```python
from build123d import *

# Parameters (mm, degrees)
SKETCH1_W                      = 300
SKETCH1_H                      = 350
BASE_FLANGE1_DEPTH             = 0.9
EDGE_FLANGE1_STRIP_W           = 5.4
EDGE_FLANGE1_STRIP_H           = 0.9
EDGE_FLANGE1_STRIP_CUT_DEPTH   = 350
EDGE_FLANGE1_STRIP_2_W         = 5.4
EDGE_FLANGE1_STRIP_2_H         = 0.9
EDGE_FLANGE1_STRIP_CUT_2_DEPTH = 350
EDGE_FLANGE1_DEPTH             = 350
EDGE_FLANGE1_BEND_DEPTH        = 350
EDGE_FLANGE2_STRIP_W           = 5.4
EDGE_FLANGE2_STRIP_H           = 0.9
EDGE_FLANGE2_STRIP_CUT_DEPTH   = 350
EDGE_FLANGE2_STRIP_2_W         = 5.4
EDGE_FLANGE2_STRIP_2_H         = 0.9
EDGE_FLANGE2_STRIP_CUT_2_DEPTH = 350
EDGE_FLANGE2_DEPTH             = 350
EDGE_FLANGE2_BEND_DEPTH        = 350
EDGE_FLANGE3_STRIP_W           = 5.4
EDGE_FLANGE3_STRIP_H           = 0.9
EDGE_FLANGE3_STRIP_CUT_DEPTH   = 350
EDGE_FLANGE3_STRIP_2_W         = 5.4
EDGE_FLANGE3_STRIP_2_H         = 0.9
EDGE_FLANGE3_STRIP_CUT_2_DEPTH = 350
EDGE_FLANGE3_DEPTH             = 350
EDGE_FLANGE3_BEND_DEPTH        = 350
CUT_EXTRUDE1_START             = 160
CUT_EXTRUDE1_DEPTH             = 15
MIRROR2_START                  = 160
MIRROR2_COPY_1_DEPTH           = 15
EDGE_FLANGE4_STRIP_W           = 5.4
EDGE_FLANGE4_STRIP_H           = 0.9
EDGE_FLANGE4_STRIP_CUT_DEPTH   = 320
EDGE_FLANGE4_DEPTH             = 320
SKETCH28_R                     = 3
CUT_EXTRUDE2_DEPTH             = 10


# Read off the part's stored shape, not the designer's step: Cut-Extrude1
# Sheet-metal steps are written as plain solids
with BuildPart() as part:
    # Sketch1 → Base-Flange1 (new body)
    with BuildSketch(Plane.XY):
        Rectangle(SKETCH1_W, SKETCH1_H)
    extrude(amount=-BASE_FLANGE1_DEPTH)

    # Edge-Flange1 strip (across the edge) → Edge-Flange1 strip cut (cut)
    with BuildSketch(Plane(origin=(-150, 175, 0), x_dir=(1, 0, 0), z_dir=(0, -1, 0))):
        with Locations((-0.9, -0.45)):
            Rectangle(EDGE_FLANGE1_STRIP_W, EDGE_FLANGE1_STRIP_H)
    extrude(amount=EDGE_FLANGE1_STRIP_CUT_DEPTH, mode=Mode.SUBTRACT)

    # Edge-Flange1 strip 2 (across the edge) → Edge-Flange1 strip cut 2 (cut)
    with BuildSketch(Plane(origin=(150, -175, 0), x_dir=(-1, 0, 0), z_dir=(0, 1, 0))):
        with Locations((-0.9, -0.45)):
            Rectangle(EDGE_FLANGE1_STRIP_2_W, EDGE_FLANGE1_STRIP_2_H)
    extrude(amount=EDGE_FLANGE1_STRIP_CUT_2_DEPTH, mode=Mode.SUBTRACT)

    # Edge-Flange1 section (across the edge) → Edge-Flange1 (add)
    with BuildSketch(Plane(origin=(-150, 175, 0), x_dir=(1, 0, 0), z_dir=(0, -1, 0))):
        with BuildLine():
            Line((0, 0.9), (0, 199.1))
            Line((0, 199.1), (0.9, 199.1))
            Line((0.9, 199.1), (0.9, 0.9))
            ThreePointArc((0.9, 0.9), (1.163603897, 0.263603897), (1.8, 0))
            Line((1.8, 0), (1.8, -0.9))
            ThreePointArc((1.8, -0.9), (0.527207794, -0.372792206), (0, 0.9))
        make_face()
    extrude(amount=EDGE_FLANGE1_DEPTH)

    # Edge-Flange1 section 2 (across the edge) → Edge-Flange1 bend (add)
    with BuildSketch(Plane(origin=(150, -175, 0), x_dir=(-1, 0, 0), z_dir=(0, 1, 0))):
        with BuildLine():
            Line((0, 0.9), (0, 199.1))
            Line((0, 199.1), (0.9, 199.1))
            Line((0.9, 199.1), (0.9, 0.9))
            ThreePointArc((0.9, 0.9), (1.163603897, 0.263603897), (1.8, 0))
            Line((1.8, 0), (1.8, -0.9))
            ThreePointArc((1.8, -0.9), (0.527207794, -0.372792206), (0, 0.9))
        make_face()
    extrude(amount=EDGE_FLANGE1_BEND_DEPTH)

    # Edge-Flange2 strip (across the edge) → Edge-Flange2 strip cut (cut)
    with BuildSketch(Plane(origin=(-149.1, 175, 199.1), x_dir=(0, 0, -1), z_dir=(0, -1, 0))):
        with Locations((-0.9, -0.45)):
            Rectangle(EDGE_FLANGE2_STRIP_W, EDGE_FLANGE2_STRIP_H)
    extrude(amount=EDGE_FLANGE2_STRIP_CUT_DEPTH, mode=Mode.SUBTRACT)

    # Edge-Flange2 strip 2 (across the edge) → Edge-Flange2 strip cut 2 (cut)
    with BuildSketch(Plane(origin=(149.1, -175, 199.1), x_dir=(0, 0, -1), z_dir=(0, 1, 0))):
        with Locations((-0.9, -0.45)):
            Rectangle(EDGE_FLANGE2_STRIP_2_W, EDGE_FLANGE2_STRIP_2_H)
    extrude(amount=EDGE_FLANGE2_STRIP_CUT_2_DEPTH, mode=Mode.SUBTRACT)

    # Edge-Flange2 section (across the edge) → Edge-Flange2 (add)
    with BuildSketch(Plane(origin=(-149.1, 175, 199.1), x_dir=(0, 0, -1), z_dir=(0, -1, 0))):
        with BuildLine():
            Line((0, 0.9), (0, 19.1))
            Line((0, 19.1), (0.9, 19.1))
            Line((0.9, 19.1), (0.9, 0.9))
            ThreePointArc((0.9, 0.9), (1.163603897, 0.263603897), (1.8, 0))
            Line((1.8, 0), (1.8, -0.9))
            ThreePointArc((1.8, -0.9), (0.527207794, -0.372792206), (0, 0.9))
        make_face()
    extrude(amount=EDGE_FLANGE2_DEPTH)

    # Edge-Flange2 section 2 (across the edge) → Edge-Flange2 bend (add)
    with BuildSketch(Plane(origin=(149.1, -175, 199.1), x_dir=(0, 0, -1), z_dir=(0, 1, 0))):
        with BuildLine():
            Line((0, 0.9), (0, 19.1))
            Line((0, 19.1), (0.9, 19.1))
            Line((0.9, 19.1), (0.9, 0.9))
            ThreePointArc((0.9, 0.9), (1.163603897, 0.263603897), (1.8, 0))
            Line((1.8, 0), (1.8, -0.9))
            ThreePointArc((1.8, -0.9), (0.527207794, -0.372792206), (0, 0.9))
        make_face()
    extrude(amount=EDGE_FLANGE2_BEND_DEPTH)

    # Edge-Flange3 strip (across the edge) → Edge-Flange3 strip cut (cut)
    with BuildSketch(Plane(origin=(130, -175, 198.2), x_dir=(1, 0, 0), z_dir=(0, 1, 0))):
        with Locations((-0.9, -0.45)):
            Rectangle(EDGE_FLANGE3_STRIP_W, EDGE_FLANGE3_STRIP_H)
    extrude(amount=EDGE_FLANGE3_STRIP_CUT_DEPTH, mode=Mode.SUBTRACT)

    # Edge-Flange3 strip 2 (across the edge) → Edge-Flange3 strip cut 2 (cut)
    with BuildSketch(Plane(origin=(-130, 175, 198.2), x_dir=(-1, 0, 0), z_dir=(0, -1, 0))):
        with Locations((-0.9, -0.45)):
            Rectangle(EDGE_FLANGE3_STRIP_2_W, EDGE_FLANGE3_STRIP_2_H)
    extrude(amount=EDGE_FLANGE3_STRIP_CUT_2_DEPTH, mode=Mode.SUBTRACT)

    # Edge-Flange3 section (across the edge) → Edge-Flange3 (add)
    with BuildSketch(Plane(origin=(130, -175, 198.2), x_dir=(1, 0, 0), z_dir=(0, 1, 0))):
        with BuildLine():
            Line((0, 0.9), (0, 19.1))
            Line((0, 19.1), (0.9, 19.1))
            Line((0.9, 19.1), (0.9, 0.9))
            ThreePointArc((0.9, 0.9), (1.163603897, 0.263603897), (1.8, 0))
            Line((1.8, 0), (1.8, -0.9))
            ThreePointArc((1.8, -0.9), (0.527207794, -0.372792206), (0, 0.9))
        make_face()
    extrude(amount=EDGE_FLANGE3_DEPTH)

    # Edge-Flange3 section 2 (across the edge) → Edge-Flange3 bend (add)
    with BuildSketch(Plane(origin=(-130, 175, 198.2), x_dir=(-1, 0, 0), z_dir=(0, -1, 0))):
        with BuildLine():
            Line((0, 0.9), (0, 19.1))
            Line((0, 19.1), (0.9, 19.1))
            Line((0.9, 19.1), (0.9, 0.9))
            ThreePointArc((0.9, 0.9), (1.163603897, 0.263603897), (1.8, 0))
            Line((1.8, 0), (1.8, -0.9))
            ThreePointArc((1.8, -0.9), (0.527207794, -0.372792206), (0, 0.9))
        make_face()
    extrude(amount=EDGE_FLANGE3_BEND_DEPTH)

    # Cut-Extrude1 outline → Cut-Extrude1 (cut)
    with BuildSketch(Plane(origin=(0, 0, 0), x_dir=(1, 0, 0), z_dir=(0, 1, 0)).offset(CUT_EXTRUDE1_START)):
        with BuildLine():
            ThreePointArc((-148.2, -198.2), (-148.836396103, -197.936396103), (-149.1, -197.3))
            Line((-149.1, -197.3), (-150, -197.3))
            ThreePointArc((-150, -197.3), (-149.472792206, -198.572792206), (-148.2, -199.1))
            Line((-148.2, -199.1), (-131.8, -199.1))
            ThreePointArc((-131.8, -199.1), (-130.527207794, -198.572792206), (-130, -197.3))
            Line((-130, -197.3), (-130, -179.1))
            Line((-130, -179.1), (-130.9, -179.1))
            Line((-130.9, -179.1), (-130.9, -197.3))
            ThreePointArc((-130.9, -197.3), (-131.163603897, -197.936396103), (-131.8, -198.2))
            Line((-131.8, -198.2), (-148.2, -198.2))
        make_face()
    cut_extrude1 = extrude(amount=CUT_EXTRUDE1_DEPTH, mode=Mode.SUBTRACT)

    # Mirror1: Cut-Extrude1 across plane
    add(cut_extrude1.mirror(Plane(origin=(0, 0, 0), x_dir=(0, 0, 1), z_dir=(1, 0, 0))), mode=Mode.SUBTRACT)

    # Mirror2: Cut-Extrude1 across plane
    add(cut_extrude1.mirror(Plane.ZX), mode=Mode.SUBTRACT)

    # Mirror2 copy 1 sketch → Mirror2 copy 1 (cut)
    with BuildSketch(Plane(origin=(0, 0, 0), x_dir=(-1, 0, 0), z_dir=(0, -1, 0)).offset(MIRROR2_START)):
        with BuildLine():
            ThreePointArc((-148.2, -198.2), (-148.836396103, -197.936396103), (-149.1, -197.3))
            Line((-149.1, -197.3), (-150, -197.3))
            ThreePointArc((-150, -197.3), (-149.472792206, -198.572792206), (-148.2, -199.1))
            Line((-148.2, -199.1), (-131.8, -199.1))
            ThreePointArc((-131.8, -199.1), (-130.527207794, -198.572792206), (-130, -197.3))
            Line((-130, -197.3), (-130, -179.1))
            Line((-130, -179.1), (-130.9, -179.1))
            Line((-130.9, -179.1), (-130.9, -197.3))
            ThreePointArc((-130.9, -197.3), (-131.163603897, -197.936396103), (-131.8, -198.2))
            Line((-131.8, -198.2), (-148.2, -198.2))
        make_face()
    extrude(amount=MIRROR2_COPY_1_DEPTH, mode=Mode.SUBTRACT)

    # Edge-Flange4 strip (across the edge) → Edge-Flange4 strip cut (cut)
    with BuildSketch(Plane(origin=(130, 160, 179.1), x_dir=(0, 0, 1), z_dir=(0, -1, 0))):
        with Locations((-1.8, -0.45)):
            Rectangle(EDGE_FLANGE4_STRIP_W, EDGE_FLANGE4_STRIP_H)
    extrude(amount=EDGE_FLANGE4_STRIP_CUT_DEPTH, mode=Mode.SUBTRACT)

    # Edge-Flange4 section (across the edge) → Edge-Flange4 (add)
    with BuildSketch(Plane(origin=(130, 160, 179.1), x_dir=(0, 0, 1), z_dir=(0, -1, 0))):
        with BuildLine():
            Line((-0.9, 0.9), (-0.9, 14.1))
            Line((-0.9, 14.1), (0, 14.1))
            Line((0, 14.1), (0, 0.9))
            ThreePointArc((0, 0.9), (0.263603897, 0.263603897), (0.9, 0))
            Line((0.9, 0), (0.9, -0.9))
            ThreePointArc((0.9, -0.9), (-0.372792206, -0.372792206), (-0.9, 0.9))
        make_face()
    extrude(amount=EDGE_FLANGE4_DEPTH)

    # Sketch28 → Cut-Extrude2 (cut)
    with BuildSketch(Plane(origin=(0, 0, -0.9), x_dir=(-1, 0, 0), z_dir=(0, 0, -1))):
        with Locations((0, 150)):
            Circle(SKETCH28_R)
        with Locations((0, -150)):
            Circle(SKETCH28_R)
    extrude(amount=-CUT_EXTRUDE2_DEPTH, mode=Mode.SUBTRACT)


solid = part.part
```
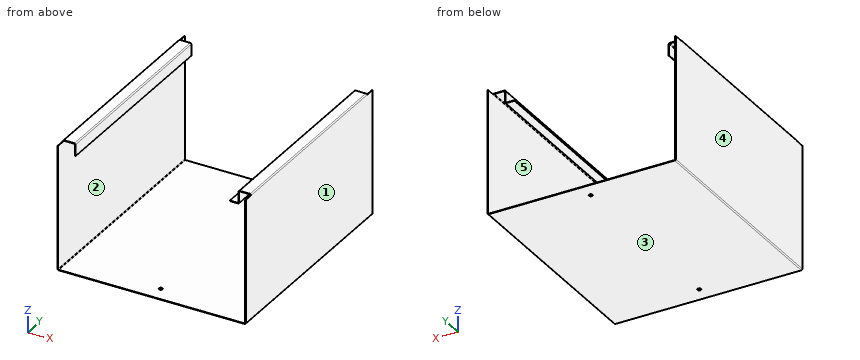
The listing builds one solid part. Answer for the finished solid, in the listing's coordinates (mm). Face numbers are marked on the shaded views. A direction names the side the tool comes from. Give positions to 0.01 mm unless a question says otherwise; leave off trailing zeros. Loops run counter-clockwise (first coordinate to the right, second up) from the corner with the lowest first, then second, coordinate; pieces in that order, holes last. Notation, with made-up numbers: (68.25, 83.25) - (87.25, 83.25) arc R26 ccw to (87.25, 112.25) - close; hole circle Ø4 at (72, -38.5). An arc over 180 degrees is marked (long way). Return JSON: item names as keys, results as strings. Group by question number.
1. Which of the six approach directions +Z, -Z, +X, -X, +Y, -Y give full straight-line access (tool end or side, diameter ignored) to the marked faces 4 and 5?
2. Given pin 1 Ø6.5 at (x, y) = (121, 1.5) entering from +Z; pin 2 Ø10.5 at (x, z) = (138, 191.5) entering from +Y; pin 3 Ø1 at (x, y) = (149.5, 166.5) entering from +Z; pin 4 Ø12 at (x, y) = (-15.5, 108.5) entering from +Z, each flat-ended and moving along its own axis, determine where each tip first touches the part or whether it passes through.
3. Straight lines are drawn through the part: line 1 (X direction, y = 9, z = 119); line 2 (Y direction, x = 0, z = -0.2); line 3 (Z direction, x = -137, y = -131.5). For each, find the intervals that lie inside material, in ascending order. Write a range as [from, to].
4. Determine the mould class of the marked faces 1, 2 and 3 for opening direction Z: pulls with the +Z half, pulls with the -Z half, needs draft (parallel to the pull), parting line crosses it, or undercut.
5. Find section C-C (x = 64). Write down the section's boundary in (y, z), then the cut area to 3 significant figures.
6. Find section A-A (z = 24). Write down the section's boundary in (x, y).
Verdict:
{
 "1": {"face 4": "+Z, -Z, -X, +Y, -Y", "face 5": "+Y, -Y"},
 "2": {"pin 1": "stops at z = 179.1", "pin 2": "passes through", "pin 3": "stops at z = 197.3", "pin 4": "stops at z = 0"},
 "3": {"line 1": "x = [-150, -149.1], [149.1, 150]", "line 2": "y = [-175, -153], [-147, 147], [153, 175]", "line 3": "z = [-0.9, 0], [198.2, 199.1]"},
 "4": {"face 1": "needs draft", "face 2": "undercut", "face 3": "pulls with the -Z half"},
 "5": {"outline": "(-175, -0.9) - (175, -0.9) - (175, 0) - (-175, 0) - close", "area": "315 mm^2"},
 "6": {"outline": "(-150, -175) - (-149.1, -175) - (-149.1, 175) - (-150, 175) - close; (149.1, -175) - (150, -175) - (150, 175) - (149.1, 175) - close"}
}
